from build123d import *

# Parameters (mm, degrees)
SKETCH_1_R          = 1.5
EXTRUDE_1_DEPTH     = 4
FILLET_2_R          = 5
CUT_EXTRUDE_1_DEPTH = 5
FILLET_3_R          = 5
FILLET_4_R          = 2


with BuildPart() as part:
    # 草图1 → 凸台-拉伸1 (new body)
    with BuildSketch(Plane.XY):
        with BuildLine():
            Line((12.667454416, 18.14297047), (-5.445003471, 4.494254472))
            Line((-5.445003471, 4.494254472), (-17.69465686, 2.402060789))
            ThreePointArc((-17.69465686, 2.402060789), (-20.647536301, -0.032105177), (-21.014322116, -3.841321514))
            Line((-21.014322116, -3.841321514), (-18.090605069, -13.404369074))
            ThreePointArc((-18.090605069, -13.404369074), (-15.656439103, -16.357248515), (-11.847222766, -16.72403433))
            Line((-11.847222766, -16.72403433), (29.431618129, -4.103826174))
            Line((29.431618129, -4.103826174), (12.667454416, 18.14297047))
        make_face()
        with Locations((11.05402554, 11.9758622)):
            Circle(SKETCH_1_R, mode=Mode.SUBTRACT)
        with Locations((4.66494146, 7.161342014)):
            Circle(SKETCH_1_R, mode=Mode.SUBTRACT)
        with Locations((-16.238278615, -1.335446723)):
            Circle(SKETCH_1_R, mode=Mode.SUBTRACT)
        with Locations((-1.254161086, -9.302643338)):
            Circle(SKETCH_1_R, mode=Mode.SUBTRACT)
    extrude(amount=EXTRUDE_1_DEPTH)

    # 圆角2
    fillet_2_edges = [part.edges().sort_by_distance(p)[0] for p in [
        (-5.445003471, 4.494254472, 2),
        (12.667454416, 18.14297047, 2),
    ]]
    fillet(fillet_2_edges, radius=FILLET_2_R)

    # 草图2 → 切除-拉伸1 (cut, through all)
    with BuildSketch(Plane(origin=(0, 0, 0), x_dir=(-1, 0, 0), z_dir=(0, 0, -1))):
        Polygon((-19.802577759, 8.674341987), (-3.664326363, -11.981677845), (-29.431618129, -4.103826174), align=None)
    extrude(amount=-CUT_EXTRUDE_1_DEPTH, mode=Mode.SUBTRACT)

    # 圆角3
    fillet_3_edges = [part.edges().sort_by_distance(p)[0] for p in [
        (19.802577759, 8.674341987, 2),
        (3.664326363, -11.981677845, 2),
    ]]
    fillet(fillet_3_edges, radius=FILLET_3_R)

    # 圆角4
    fillet_4_edges = [part.edges().sort_by_distance(p)[0] for p in [
        (-17.69465686, 2.402060789, 2),
    ]]
    fillet(fillet_4_edges, radius=FILLET_4_R)


solid = part.part
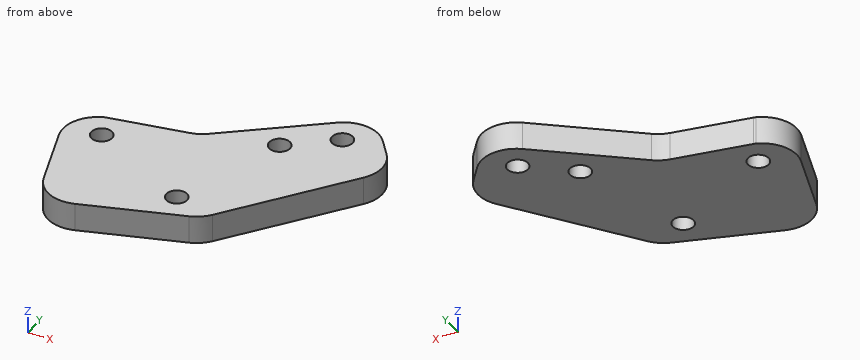
Here's how the part is built. I have some questions about the finished solid (model axes, mm). Coordinates: 2 decimals unless noted, no trailing zeros. Order: outer loops, then holes, each group sorted by start corner. A loop starts at its lowest first (then second) coordinate and runs counter-clockwise, first axis right, second up. Notation, with made-up numbers: (67, 32.25) -> (126, 32.25) arc R10 cw to (126, 49.25) -> close; hole circle Ø11 at (45.25, 15). An arc over 180 degrees is marked (long way). Answer in a Markdown table with one row per item.
(1) I want a section at B-B on x = -16. List the corners of the cut face in (y, z) for me.
Answer key:
| item | result |
|---|---|
| outline | (-16.16, 0) -> (-2.82, 0) -> (-2.82, 4) -> (-16.16, 4) -> close; (0.15, 0) -> (2.69, 0) -> (2.69, 4) -> (0.15, 4) -> close |
(2) I want a section at D-D on x = 13. List the corners of the cut face in (y, z) for me.
Answer key:
| item | result |
|---|---|
| outline | (-0.03, 0) -> (15.96, 0) -> (15.96, 4) -> (-0.03, 4) -> close |
(3) I want a section at A-A on z = 1.8. List the corners of the cut face in (x, y) for me, then the cut area to 3 significant figures.
Answer key:
| item | result |
|---|---|
| outline | (-21.01, -3.84) -> (-18.09, -13.4) arc R5 ccw to (-11.85, -16.72) -> (2.16, -12.44) arc R5 ccw to (4.63, -10.74) -> (17.44, 5.65) arc R5 ccw to (17.49, 11.74) -> (15.68, 14.15) arc R5 ccw to (8.67, 15.13) -> (-4.47, 5.23) arc R5 cw to (-6.64, 4.29) -> (-17.55, 2.43) arc R2 ccw to (-17.87, 2.34) arc R5 ccw to start; hole circle Ø3 at (-16.24, -1.34); hole circle Ø3 at (-1.25, -9.3); hole circle Ø3 at (4.66, 7.16); hole circle Ø3 at (11.05, 11.98) |
| area | 687 mm^2 |
(4) Please list where these lines run through material, in increasing order: probe 1 along X at (y, z) = (-2.5, 2.75); probe 2 along X at (y, z) = (11.5, 2.6); probe 3 along Y at (x, z) = (4.5, 2.15).
Answer key:
| item | result |
|---|---|
| probe 1 | -21.23 to -17.18, -15.29 to 11.07 |
| probe 2 | 3.85 to 9.63, 12.48 to 17.66 |
| probe 3 | -10.9 to 5.67, 8.65 to 11.99 |
(5) Will these pins go through, and if not, where does the flat tip stop? pin 1 Ø2 at (x, z) = (3, 1.5) entering from +Y; pin 2 Ø1.8 at (x, y) = (-16.24, -1.34) entering from -Z; pin 3 Ø1 at (y, z) = (-10, 0.5) entering from +X.
Answer key:
| item | result |
|---|---|
| pin 1 | y = 11.61 |
| pin 2 | through |
| pin 3 | x = 5.6 |
(6) I want a section at C-C on y = 13. List the corners of the cut face in (x, z) for me.
Answer key:
| item | result |
|---|---|
| outline | (5.84, 0) -> (9.96, 0) -> (9.96, 4) -> (5.84, 4) -> close; (12.15, 0) -> (16.54, 0) -> (16.54, 4) -> (12.15, 4) -> close |
